The listing builds one solid part. Answer for the finished solid, in the listing's coordinates (mm). Face numbers are marked on the shaded views. A direction names the side the tool comes from. Give positions to 0.01 mm unless a question says otherwise; leave off trailing zeros. Order: outer loops, then holes, each group sorted by start corner. A loop starts at its lowest first (then second) coordinate and runs counter-clockwise, first axis right, second up. Notation, with made-up numbers: (89.5, 9) - (143.5, 9) arc R24 ccw to (143.5, 22) - close; hole circle Ø7 at (36, 55.25). An arc over 180 degrees is marked (long way). Answer as a JSON object with one key per item and string values. Group by question number.
Q1. A cutting plane is placed at C-C, the plane x = -1.5. Give the vertices of the cut face in (y, z), and give its area (3 significant figures).
Q2. Consider line 1 (Z direction, x = -18, y = 0); line 2 (Z direction, x = -16, y = 23); line 3 (Y direction, x = 7.5, z = 2.5). Determine where each line is inside the solid, lowest interval first.
Q3. Given pin 1 (3 mm diameter, centred on x = -13, y = -34.5, fed in from -Z); pin 2 (1.5 mm diameter, centred on x = 8, y = -30, fed in from +Z); pin 3 (2 mm diameter, centred on y = -28, z = 26, fed in from +X); pin 4 (12 mm diameter, centred on y = -29, z = -27.5, fed in from -X), each flat-ended and moving along its own axis, determine where each tip first touches the part or whether it passes through.
Q4. A cutting plane is placed at D-D, the plane z = 16. Give the vertices of the cut face in (x, y).
Q5. For the marked faces 1 and 2, determine the directions among +Z, -Z, +X, -X, +Y, -Y from which every point of the face is accessible in a straight line to the end or side of a thin tool.
Q6. The mould has two halves that part along Z. Classify the marked faces 3, 4, 5 and 6: released by +Z, released by -Z, zero draft, split by the parting line, or undercut.
Q7. A cutting plane is placed at A-A, the plane z = 0. Give the vertices of the cut face in (x, y).
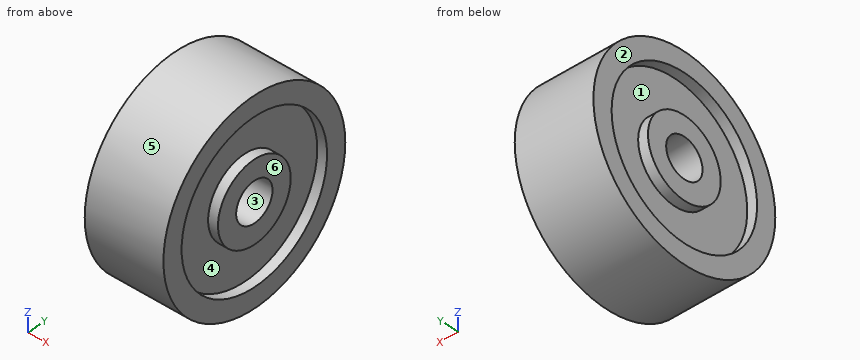
Autodesk Inventor part; units mm, degrees
ref_plane "YZ Plane" through (0, 0, 0) normal (1, 0, 0) x (0, 1, 0)
ref_plane "XZ Plane" through (0, 0, 0) normal (0, 1, 0) x (-1, 0, 0)
ref_plane "XY Plane" through (0, 0, 0) normal (0, 0, 1) x (1, 0, 0)
sketch "Esboço1" plane through (0, 0, 0) normal (1, 0, 0) x (0, 1, 0)
  circle A0 centre (0, 0) radius 50
  circle A1 centre (0, 0) radius 40
  circle A2 centre (0, 0) radius 10
  circle A3 centre (0, 0) radius 20
extrude "Extrusão1" add sketch "Esboço1" along normal mid plane 40
sketch "Esboço3" plane through (0, 0, 0) normal (1, 0, 0) x (0, 1, 0)
  circle A0 centre (0, 0) radius 20
  circle A1 centre (0, 0) radius 40
extrude "Extrusão2" add sketch "Esboço3" along normal mid plane 30
Reply:
{
 "1": {"outline": "circle Ø100 at (0, 0); hole circle Ø20 at (0, 0)", "area": "7,540 mm^2"},
 "2": {"line 1": "z = -50 to -40, -20 to -10, 10 to 20, 40 to 50", "line 2": "z = -44.4 to -32.73, 32.73 to 44.4", "line 3": "y = -49.94 to -9.68, 9.68 to 49.94"},
 "3": {"pin 1": "stops at z = -37.56", "pin 2": "stops at z = 40.55", "pin 3": "stops at x = 15", "pin 4": "stops at x = -20"},
 "4": {"outline": "(-20, -47.37) - (20, -47.37) - (20, -36.66) - (15, -36.66) - (15, -12) - (20, -12) - (20, 12) - (15, 12) - (15, 36.66) - (20, 36.66) - (20, 47.37) - (-20, 47.37) - (-20, 36.66) - (-15, 36.66) - (-15, 12) - (-20, 12) - (-20, -12) - (-15, -12) - (-15, -36.66) - (-20, -36.66) - close"},
 "5": {"face 1": "-X", "face 2": "+Z, -Z, -X, +Y, -Y"},
 "6": {"face 3": "undercut", "face 4": "undercut", "face 5": "split by the parting line", "face 6": "zero draft"},
 "7": {"outline": "(-20, -50) - (20, -50) - (20, -40) - (15, -40) - (15, -20) - (20, -20) - (20, -10) - (-20, -10) - (-20, -20) - (-15, -20) - (-15, -40) - (-20, -40) - close; (-20, 10) - (20, 10) - (20, 20) - (15, 20) - (15, 40) - (20, 40) - (20, 50) - (-20, 50) - (-20, 40) - (-15, 40) - (-15, 20) - (-20, 20) - close"}
}
